Geometry check sheet. Reference: the model listing, model coordinates, mm. Face numbers are marked on the shaded views. A direction names the side the tool comes from. Coordinates: 2 decimals unless noted, no trailing zeros. Loops run counter-clockwise (first coordinate to the right, second up) from the corner with the lowest first, then second, coordinate; pieces in that order, holes last. Notation, with made-up numbers: M 19,71.25 L 68,71.25 A26 ccw 68,102.25 Z; hole C 42.5,-34 d9. An arc over 180 degrees is marked long. Use CSV: the item, a comma, the result in double quotes.
```python
from build123d import *

# Parameters (mm, degrees)
SKETCH1_W           = 55.6
SKETCH1_H           = 55.6
BOSS_EXTRUDE1_DEPTH = 23.1
FILLET1_R           = 10
SKETCH2_R           = 1
SCREW_HOLES_DEPTH   = 4
SKETCH3_R           = 26.5
BOSS_EXTRUDE2_DEPTH = 18.2
CHAMFER1_SIZE       = 3


with BuildPart() as part:
    # Sketch1 → Boss-Extrude1 (new body)
    with BuildSketch(Plane(origin=(0, 0, 0), x_dir=(1, 0, 0), z_dir=(0, 1, 0))):
        with Locations((27.8, 27.8)):
            Rectangle(SKETCH1_W, SKETCH1_H)
    extrude(amount=BOSS_EXTRUDE1_DEPTH)

    # Fillet1
    fillet1_edges = [part.edges().sort_by_distance(p)[0] for p in [
        (0, 11.55, -55.6),
        (55.6, 11.55, -55.6),
        (55.6, 11.55, 0),
        (0, 11.55, 0),
    ]]
    fillet(fillet1_edges, radius=FILLET1_R)

    # Sketch2 → Screw Holes (cut)
    with BuildSketch(Plane.XZ):
        with Locations(Location((6.3, -6.3, 0), (0, 0, 270))):
            Circle(SKETCH2_R)
        with Locations(Location((49.3, -6.3, 0), (0, 0, 270))):
            Circle(SKETCH2_R)
        with Locations(Location((49.3, -49.3, 0), (0, 0, 270))):
            Circle(SKETCH2_R)
        with Locations(Location((6.3, -49.3, 0), (0, 0, 270))):
            Circle(SKETCH2_R)
    extrude(amount=-SCREW_HOLES_DEPTH, mode=Mode.SUBTRACT)

    # Sketch3 → Boss-Extrude2 (add)
    with BuildSketch(Plane(origin=(0, 23.1, 0), x_dir=(1, 0, 0), z_dir=(0, 1, 0))):
        with Locations(Location((27.8, 27.8, 0), (0, 0, 270))):
            Circle(SKETCH3_R)
    extrude(amount=BOSS_EXTRUDE2_DEPTH)

    # Chamfer1
    chamfer1_edges = [part.edges().sort_by_distance(p)[0] for p in [
        (27.8, 41.3, -54.3),
    ]]
    chamfer(chamfer1_edges, length=CHAMFER1_SIZE)


solid = part.part
```
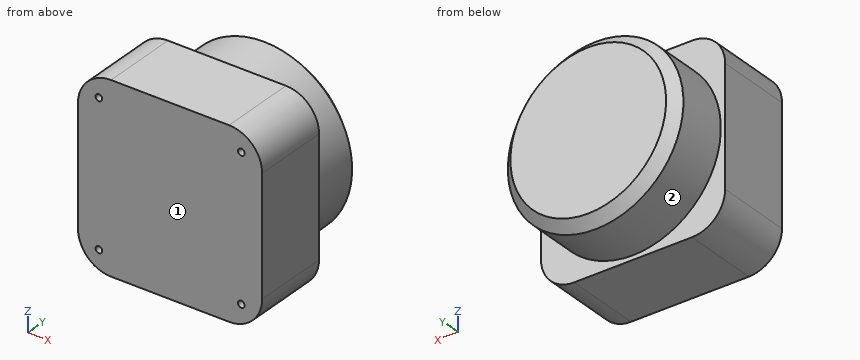
1. Section check C-C, the plane y = 24.5. Record the cut outline in (x, z).
The answers:
outline,"C 27.8,-27.8 d53"
2. Gauge pin test, flat ends, axial feed: P1, Ø1, axis at y = 29.5, z = -10.5, coming from the -X side; P2, Ø1.2, axis at x = 6.3, z = -49.3, coming from the +Y side; P3, Ø1.8, axis at x = 49.3, z = -6.3, coming from the -Y side. Record the tip position at first contact, or that the pin passes through.
The answers:
P1,"x = 7.31"
P2,"y = 23.1"
P3,"y = 4"
3. Section check A-A, the plane z = -27.8. Record the cut outline in (x, y).
The answers:
outline,"M 0,0 L 55.6,0 L 55.6,23.1 L 54.3,23.1 L 54.3,38.3 L 51.3,41.3 L 4.3,41.3 L 1.3,38.3 L 1.3,23.1 L 0,23.1 Z"
4. Thickness scan on line 1 (Z direction, x = 6, y = 1); line 2 (X direction, y = 1.05, z = -6.3); line 3 (Z direction, x = 49, y = 2). Record the ranges inside material, lowest first. Write a range as [from, to].
The answers:
line 1,"[-54.77, -50.25], [-48.35, -7.25], [-5.35, -0.83]"
line 2,"[0.71, 5.3], [7.3, 48.3], [50.3, 54.89]"
line 3,"[-55, -50.25], [-48.35, -7.25], [-5.35, -0.6]"
5. Section check B-B, the plane y = 18. Record the cut outline in (x, z).
The answers:
outline,"M 0,-45.6 A10 ccw 10,-55.6 L 45.6,-55.6 A10 ccw 55.6,-45.6 L 55.6,-10 A10 ccw 45.6,0 L 10,0 A10 ccw 0,-10 Z"
6. Set-up check for the marked faces 1 and 2: record each of +Z, -Z, +X, -X, +Y, -Y from which the full face is reachable in a straight line by a thin tool's end or side.
The answers:
face 1,"+Z, -Z, +X, -X, -Y"
face 2,"+Y"
